Here's how the part is built. I have some questions about the finished solid (model axes, mm). Give positions to 0.01 mm unless a question says otherwise; leave off trailing zeros. Loops run counter-clockwise (first coordinate to the right, second up) from the corner with the lowest first, then second, coordinate; pieces in that order, holes last. Notation, with made-up numbers: (-24, -18.5) - (19, -18.5) arc R29 ccw to (19, 5.5) - close; hole circle Ø6 at (26.5, 62). An arc over 180 degrees is marked (long way). Put each result on its own line as item: value. Start each with the question number.
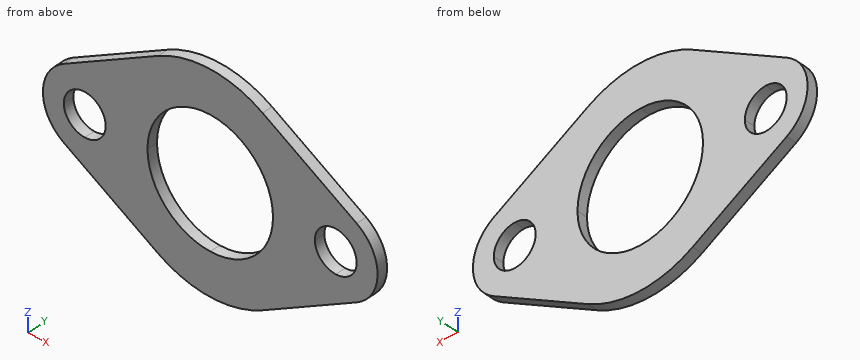
from build123d import *

# Parameters (mm, degrees)
F1_DEPTH = 1.5748


with BuildPart() as f1:
    # F0 (on Front) → F1 (new body)
    with BuildSketch(Plane.XZ):
        with BuildLine():
            Line((-7.9375, 13.748153), (-22.225, 5.499261))
            ThreePointArc((-22.225, 5.499261), (-25.4, 0), (-22.225, -5.499261))
            Line((-22.225, -5.499261), (-7.9375, -13.748153))
            ThreePointArc((-7.9375, -13.748153), (0, -15.875), (7.9375, -13.748153))
            Line((7.9375, -13.748153), (22.225, -5.499261))
            ThreePointArc((22.225, -5.499261), (25.4, 0), (22.225, 5.499261))
            Line((22.225, 5.499261), (7.9375, 13.748153))
            ThreePointArc((7.9375, 13.748153), (0, 15.875), (-7.9375, 13.748153))
        make_face()
        with BuildLine():
            ThreePointArc((-19.05, 3.175), (-16.804936, 2.245064), (-15.875, 0))
            ThreePointArc((-15.875, 0), (-16.804936, -2.245064), (-19.05, -3.175))
            ThreePointArc((-19.05, -3.175), (-21.295064, -2.245064), (-22.225, 0))
            ThreePointArc((-22.225, 0), (-21.295064, 2.245064), (-19.05, 3.175))
        make_face(mode=Mode.SUBTRACT)
        with BuildLine():
            ThreePointArc((0, 9.525), (6.735192, 6.735192), (9.525, 0))
            ThreePointArc((9.525, 0), (6.735192, -6.735192), (0, -9.525))
            ThreePointArc((0, -9.525), (-6.735192, -6.735192), (-9.525, 0))
            ThreePointArc((-9.525, 0), (-6.735192, 6.735192), (0, 9.525))
        make_face(mode=Mode.SUBTRACT)
        with BuildLine():
            ThreePointArc((19.05, 3.175), (21.295064, 2.245064), (22.225, 0))
            ThreePointArc((22.225, 0), (21.295064, -2.245064), (19.05, -3.175))
            ThreePointArc((19.05, -3.175), (16.804936, -2.245064), (15.875, 0))
            ThreePointArc((15.875, 0), (16.804936, 2.245064), (19.05, 3.175))
        make_face(mode=Mode.SUBTRACT)
    extrude(amount=F1_DEPTH)


solid = f1.part
1) Suppose I cut it at C-C on z = 6.5. Please give me the cut outline in (x, y), plus the area to 3 significant figures.
2) I need wall thicknesses on line 1 (X direction, y = -0.3, z = -0.5); line 2 (X direction, y = -0.3, z = 1); line 3 (X direction, y = -0.8, z = 4). Which ranges of each line are inside material? Lowest first, please.
3) Suppose I cut it at B-B on x = -6. Please give me the cut outline in (y, z).
4) I'm going to push a flat-ended pin straight in: P1, Ø5, axis at x = 6.5, z = 3.5, coming from the -Y side. Where does the tip first touch, or does it pass through?
5) Suppose I cut it at D-D on z = -1.5. Please give me the cut outline in (x, y), plus the area to 3 significant figures.
6) Suppose I cut it at A-A on y = -0.8. Give the number of separate pieces and of enclosed holes in the cut face, plus the area to 3 significant figures.
Ans:
1. outline: (-20.49, -1.57) - (-6.96, -1.57) - (-6.96, 0) - (-20.49, 0) - close; (6.96, -1.57) - (20.49, -1.57) - (20.49, 0) - (6.96, 0) - close
1. area: 42.6 mm²
2. line 1: x = -25.38 to -22.19, -15.91 to -9.51, 9.51 to 15.91, 22.19 to 25.38
2. line 2: x = -25.32 to -22.06, -16.04 to -9.47, 9.47 to 16.04, 22.06 to 25.32
2. line 3: x = -23.98 to -8.64, 8.64 to 23.98
3. outline: (-1.57, -14.7) - (0, -14.7) - (0, -7.4) - (-1.57, -7.4) - close; (-1.57, 7.4) - (0, 7.4) - (0, 14.7) - (-1.57, 14.7) - close
4. P1: stops at y = -1.57
5. outline: (-25.22, -1.57) - (-21.85, -1.57) - (-21.85, 0) - (-25.22, 0) - close; (-16.25, -1.57) - (-9.41, -1.57) - (-9.41, 0) - (-16.25, 0) - close; (9.41, -1.57) - (16.25, -1.57) - (16.25, 0) - (9.41, 0) - close; (21.85, -1.57) - (25.22, -1.57) - (25.22, 0) - (21.85, 0) - close
5. area: 32.2 mm²
6. separate pieces: 1
6. enclosed holes: 3
6. area: 733 mm²
